```python
from build123d import *

# Parameters (mm, degrees)
F1_DEPTH = 6.35
F3_R     = 1.27


# Not quite as in the source:
# - a feature of the source that left no trace in its solid (it failed there, or was rolled back) is left out


with BuildPart() as f1:
    # F0 (on Front) → F1 (new body)
    with BuildSketch(Plane.XZ):
        with BuildLine():
            ThreePointArc((0, 0), (8.8014992753, 5.1423850964), (12.1607482433, 14.766623266))
            ThreePointArc((12.1607482433, 14.766623266), (3.270966354, 9.6969414968), (0, 0))
        make_face()
    extrude(amount=F1_DEPTH)

    # F3
    f3_edges = [f1.edges().sort_by_distance(p)[0] for p in [
        (3.270966, 0, 9.696941),
        (8.801499, 0, 5.142385),
        (12.160748, -3.175, 14.766623),
        (0, -3.175, 0),
        (3.270966, -6.35, 9.696941),
        (8.801499, -6.35, 5.142385),
    ]]
    fillet(f3_edges, radius=F3_R)


solid = f1.part
```
Can you work these out from the model? Positions are in its coordinate system, mm. Coordinates: 2 decimals unless noted, no trailing zeros. Write each loop counter-clockwise with the first axis right and the second up, starting at its lowest first coordinate (ties: lowest second). Pieces come first, ordered by that corner, then holes. Notation, with made-up numbers: M 75.25,-15 L 94.25,-15 A19 ccw 94.25,13 Z; hole C 14,89.25 d7. An arc over 180 degrees is marked long. Answer as CSV lines item,"result".
Item 1: Please list where these lines run through material, in increasing order: line 1 along Z through (x, y) = (3.25, -3.25); line 2 along X through (y, z) = (-5.5, 7.75); line 3 along Z through (x, y) = (4, -5.5).
Geometry results:
line 1,"z = 0.97 to 9.67"
line 2,"x = 2 to 10.44"
line 3,"z = 1.4 to 10.41"
Item 2: I'm going to push a flat-ended pin straight in: P1, Ø1, axis at x = 7, y = -2.5, coming from the +Z side. Where does the tip first touch, or does it pass through?
Geometry results:
P1,"stops at z = 13.19"
Item 3: Imagine slicing it at A-A on y = -5.5. List the corners of the cut face in (x, z) for me.
Geometry results:
outline,"M 0.11,1.71 A1.2 ccw 1.65,0.47 A14.67 ccw 12.02,13.06 A1.2 ccw 10.5,14.33 A14.32 ccw Z"
Item 4: Imagine slicing it at B-B on y = -1. List the corners of the cut face in (x, z) for me.
Geometry results:
outline,"M 0.07,1.71 A1.24 ccw 1.66,0.43 A14.71 ccw 12.06,13.06 A1.24 ccw 10.49,14.37 A14.36 ccw Z"
